Source: CAD feature listing. Evaluate the final solid. Frame: model axes, mm. A direction names the side the tool comes from. Give positions to 0.01 mm unless a question says otherwise; leave off trailing zeros. Loops run counter-clockwise (first coordinate to the right, second up) from the corner with the lowest first, then second, coordinate; pieces in that order, holes last. Notation, with made-up numbers: (50.25, 23) -> (107.25, 23) arc R29 cw to (107.25, 47) -> close; hole circle Ø9 at (-13, -25). An arc over 180 degrees is marked (long way). Return JSON: item names as keys, results as strings. Group by question number.
```python
from build123d import *

# Parameters (mm, degrees)
SKETCH_R        = 21
PAD_DEPTH       = 4
CHAMFER_SIZE    = 0.3
CHAMFER001_SIZE = 0.3


with BuildPart() as part:
    # Sketch → Pad (new body)
    with BuildSketch(Plane.XY):
        Circle(SKETCH_R)
        Polygon((0, 17.205038), (-14.9, 8.602519), (-14.9, -8.602519), (0, -17.205038), (14.9, -8.602519), (14.9, 8.602519), align=None, mode=Mode.SUBTRACT)
    extrude(amount=PAD_DEPTH)

    # Chamfer
    chamfer_edges = [part.edges().sort_by_distance(p)[0] for p in [
        (-7.45, 12.903779, 4),
        (-14.9, 0, 4),
        (-7.45, -12.903779, 4),
        (7.45, -12.903779, 4),
        (14.9, 0, 4),
        (7.45, 12.903779, 4),
    ]]
    chamfer(chamfer_edges, length=CHAMFER_SIZE)

    # Chamfer001
    chamfer001_edges = [part.edges().sort_by_distance(p)[0] for p in [
        (-7.45, -12.903779, 0),
        (-14.9, 0, 0),
        (-7.45, 12.903779, 0),
        (7.45, 12.903779, 0),
        (14.9, 0, 0),
        (7.45, -12.903779, 0),
    ]]
    chamfer(chamfer001_edges, length=CHAMFER001_SIZE)


solid = part.part
```
1) Cut plane C-C on y = 14. Return loops of the section in (x, z).
2) Reachability of faces 1 (the face through (7.42, -13.097, 3.852)), 2 (the face through (-7.63, -12.97, 0.15)), 3 (the face through (7.35, -12.96, 1.98)) from +Z, -Z, +X, -X, +Y, -Y: full face, straight path, thin tool, end or side. Return the list, or none.
3) Cut plane D-D on x = -16. Return loops of the section in (y, z), then the cut area to 3 significant figures.
4) Contact query for flat-ended pins moving along their axis: P1, Ø1, axis at y = 1.5, z = 1.5, coming from the -X side; P2, Ø1.5, axis at y = -8.5, z = 1, coming from the +X side. Output: stop coordinate, or through.
5) Cut plane A-A on z = 2.5. Return loops of the section in (x, y), then the cut area to 3 significant figures.
6) Cut plane B-B on y = 0. Return loops of the section in (x, z), then the cut area to 3 significant figures.
7) Mould query, pull axis Y, two halves, no side actions, for faces 4 (the face through (-9.4, -12.3, 4)), 5 (the face through (20.03, 6.31, 1.97)), 6 (the face through (14.9, 0, 2)), 7 (the face through (7.554, 12.844, 1.976)). Classes: released by +Y, released by -Y, zero draft, split by the parting line, or undercut.
8) Material intervals for line 1 (X direction, y = 5.5, z = 3.35); line 2 (X direction, y = 10, z = 3.35); line 3 (Y direction, x = 2.5, z = 2.25), sorted ascending.
Calculated:
{
 "1": {"outline": "(-15.65, 0) -> (-6.15, 0) -> (-5.55, 0.3) -> (-5.55, 3.7) -> (-6.15, 4) -> (-15.65, 4) -> close; (5.55, 0.3) -> (6.15, 0) -> (15.65, 0) -> (15.65, 4) -> (6.15, 4) -> (5.55, 3.7) -> close"},
 "2": {"face 1": "+Z", "face 2": "-Z", "face 3": "+Z, -Z"},
 "3": {"outline": "(-13.6, 0) -> (13.6, 0) -> (13.6, 4) -> (-13.6, 4) -> close", "area": "109 mm2"},
 "4": {"P1": "x = -20.98", "P2": "x = 19.52"},
 "5": {"outline": "circle Ø42 at (0, 0); hole (-14.9, -8.6) -> (0, -17.21) -> (14.9, -8.6) -> (14.9, 8.6) -> (0, 17.21) -> (-14.9, 8.6) -> close", "area": "616 mm2"},
 "6": {"outline": "(-21, 0) -> (-15.2, 0) -> (-14.9, 0.3) -> (-14.9, 3.7) -> (-15.2, 4) -> (-21, 4) -> close; (14.9, 0.3) -> (15.2, 0) -> (21, 0) -> (21, 4) -> (15.2, 4) -> (14.9, 3.7) -> close", "area": "48.6 mm2"},
 "7": {"face 4": "zero draft", "face 5": "split by the parting line", "face 6": "undercut", "face 7": "undercut"},
 "8": {"line 1": "-20.27 to -14.9, 14.9 to 20.27", "line 2": "-18.47 to -12.48, 12.48 to 18.47", "line 3": "-20.85 to -15.76, 15.76 to 20.85"}
}
